Source: CAD feature listing. Evaluate the final solid. Frame: model axes, mm. A direction names the side the tool comes from. Round coordinates to 2 decimals unless told otherwise and drop trailing zeros. Write each loop counter-clockwise with the first axis right and the second up, starting at its lowest first coordinate (ties: lowest second). Pieces come first, ordered by that corner, then holes. Notation, with made-up numbers: M 5,68 L 47,68 A25 ccw 47,81 Z; hole C 32.25,8.5 d5. An arc over 180 degrees is marked long. Put each result on its own line as item: value. Start each with the question number.
```python
from build123d import *
from OCP.BRepFilletAPI import BRepFilletAPI_MakeChamfer

# Parameters (mm, degrees)
ESQUISSE1_W             = 62
ESQUISSE1_H             = 42
BOSS_EXTRU_1_DEPTH      = 15
ESQUISSE2_R             = 2.1
ESQUISSE2_R_2           = 12.5
ESQUISSE2_R_3           = 1.7
ENL_V_MAT_EXTRU_1_DEPTH = 41.33608806
ESQUISSE4_R             = 4.5
ENL_V_MAT_EXTRU_2_DEPTH = 10
SKETCH1_W               = 20
SKETCH1_H               = 42
CUT_EXTRUDE1_DEPTH      = 41.33608806
SKETCH2_W               = 15
SKETCH2_H               = 42
BOSS_EXTRUDE1_DEPTH     = 40
CUT_EXTRUDE2_DEPTH      = 68.749538744
SKETCH7_W               = 38
SKETCH7_H               = 20
CUT_EXTRUDE3_DEPTH      = 7
SKETCH9_R               = 2.1
CUT_EXTRUDE4_DEPTH      = 56.731499172
CHAMFER1_SIZE           = 38
CHAMFER1_SIZE2          = 11
SKETCH10_W              = 8
SKETCH10_H              = 24.631578948
CUT_EXTRUDE5_DEPTH      = 58.15767665
FILLET2_START           = -1
FILLET2_DEPTH           = 17
FILLET2_START_2         = -22
FILLET2_2_DEPTH         = 44
FILLET4_R               = 2
FILLET5_R               = 1


with BuildPart() as part:
    # Esquisse1 → Boss.-Extru.1 (new body)
    with BuildSketch(Plane.XY):
        Rectangle(ESQUISSE1_W, ESQUISSE1_H)
    extrude(amount=BOSS_EXTRU_1_DEPTH)

    # Esquisse2 → Enlèv. mat.-Extru.1 (cut, through all)
    with BuildSketch(Plane.XY.offset(15)):
        with Locations((21, 11)):
            Circle(ESQUISSE2_R)
        with Locations((21, -11)):
            Circle(ESQUISSE2_R)
        with Locations((-10, 0)):
            Circle(ESQUISSE2_R_2)
        with Locations((-25.5, 15.5)):
            Circle(ESQUISSE2_R_3)
        with Locations((5.5, 15.5)):
            Circle(ESQUISSE2_R_3)
        with Locations((5.5, -15.5)):
            Circle(ESQUISSE2_R_3)
        with Locations((-25.5, -15.5)):
            Circle(ESQUISSE2_R_3)
    extrude(amount=-ENL_V_MAT_EXTRU_1_DEPTH, mode=Mode.SUBTRACT)

    # Esquisse4 → Enlèv. mat.-Extru.2 (cut)
    with BuildSketch(Plane.XY.offset(15)):
        with Locations((-25.5, 15.5)):
            Circle(ESQUISSE4_R)
        with Locations((-25.5, -15.5)):
            Circle(ESQUISSE4_R)
        with Locations((5.5, -15.5)):
            Circle(ESQUISSE4_R)
        with Locations((5.5, 15.5)):
            Circle(ESQUISSE4_R)
    extrude(amount=-ENL_V_MAT_EXTRU_2_DEPTH, mode=Mode.SUBTRACT)

    # Sketch1 → Cut-Extrude1 (cut, through all)
    with BuildSketch(Plane.XY.offset(15)):
        with Locations((21, 0)):
            Rectangle(SKETCH1_W, SKETCH1_H)
    extrude(amount=-CUT_EXTRUDE1_DEPTH, mode=Mode.SUBTRACT)

    # Sketch2 → Boss-Extrude1 (add)
    with BuildSketch(Plane(origin=(11, 0, 0), x_dir=(0, 0, -1), z_dir=(1, 0, 0))):
        with Locations((-7.5, 0)):
            Rectangle(SKETCH2_W, SKETCH2_H)
    extrude(amount=BOSS_EXTRUDE1_DEPTH)

    # Sketch6 → Cut-Extrude2 (cut, through all)
    with BuildSketch(Plane.XZ.offset(21)):
        Polygon((-31, 8), (-31, 15), (13, 15), align=None)
    extrude(amount=-CUT_EXTRUDE2_DEPTH, mode=Mode.SUBTRACT)

    # Sketch7 → Cut-Extrude3 (cut)
    with BuildSketch(Plane.XY.offset(15)):
        with Locations((32, 0)):
            Rectangle(SKETCH7_W, SKETCH7_H)
    extrude(amount=-CUT_EXTRUDE3_DEPTH, mode=Mode.SUBTRACT)

    # Sketch9 → Cut-Extrude4 (cut, through all)
    with BuildSketch(Plane.XY.offset(8)):
        with Locations((21, 0)):
            Circle(SKETCH9_R)
        with Locations((35, 0)):
            Circle(SKETCH9_R)
    extrude(amount=-CUT_EXTRUDE4_DEPTH, mode=Mode.SUBTRACT)

    # Chamfer1: one chamfer whose edges measure the first distance from different faces: ONE call of the kernel's chamfer builder (chamfer() names one face for all edges)
    chamfer1_edges_1 = [part.edges().sort_by_distance(p)[0] for p in [
        (51, 21, 7.5),
    ]]
    chamfer1_side_1 = [part.faces().sort_by_distance(p)[0] for p in [
        (13.76889715, 21, 6.760532838),
    ]]
    chamfer1_edges_2 = [part.edges().sort_by_distance(p)[0] for p in [
        (51, -21, 7.5),
    ]]
    chamfer1_side_2 = [part.faces().sort_by_distance(p)[0] for p in [
        (13.76889715, -21, 6.760532838),
    ]]
    chamfer1 = BRepFilletAPI_MakeChamfer(part.part.solid().wrapped)
    for e in chamfer1_edges_1:
        chamfer1.Add(CHAMFER1_SIZE, CHAMFER1_SIZE2, e.wrapped, chamfer1_side_1[0].wrapped)  # the first distance lies on this face
    for e in chamfer1_edges_2:
        chamfer1.Add(CHAMFER1_SIZE, CHAMFER1_SIZE2, e.wrapped, chamfer1_side_2[0].wrapped)  # the first distance lies on this face
    add(Compound.cast(chamfer1.Shape()), mode=Mode.REPLACE)

    # Sketch10 → Cut-Extrude5 (cut, through all)
    with BuildSketch(Plane(origin=(0, 0, 0), x_dir=(-1, 0, 0), z_dir=(0, 0, -1))):
        with Locations((-47, 0)):
            Rectangle(SKETCH10_W, SKETCH10_H)
    extrude(amount=-CUT_EXTRUDE5_DEPTH, mode=Mode.SUBTRACT)

    # Fillet2: read off the stored shape, not the designer's step
    # Fillet2 outline → Fillet2 (cut)
    with BuildSketch(Plane.XY.offset(FILLET2_START)):
        with BuildLine():
            Line((13, 21), (10.163489291, 21))
            ThreePointArc((10.163489291, 21), (12.9718958, 20.801839634), (15.724650822, 20.211285288))
            Line((15.724650822, 20.211285288), (13, 21))
        make_face()
        with BuildLine():
            ThreePointArc((15.724650822, -20.211285288), (12.9718958, -20.801839634), (10.163489291, -21))
            Line((10.163489291, -21), (13, -21))
            Line((13, -21), (15.724650822, -20.211285288))
        make_face()
    extrude(amount=FILLET2_DEPTH, mode=Mode.SUBTRACT)

    # Fillet2 2 outline → Fillet2 2 (cut)
    with BuildSketch(Plane(origin=(0, 0, 0), x_dir=(1, 0, 0), z_dir=(0, 1, 0)).offset(FILLET2_START_2)):
        with BuildLine():
            Line((11.438667082, -14.751606127), (13, -15))
            Line((13, -15), (14.580968057, -15))
            ThreePointArc((14.580968057, -15), (13.004916429, -14.937804826), (11.438667082, -14.751606127))
        make_face()
    extrude(amount=FILLET2_2_DEPTH, mode=Mode.SUBTRACT)

    # Fillet4
    fillet4_edges = [part.edges().sort_by_distance(p)[0] for p in [
        (-31, 21, 4),
        (-31, -21, 4),
    ]]
    fillet(fillet4_edges, radius=FILLET4_R)

    # Fillet5
    fillet5_edges = [part.edges().sort_by_distance(p)[0] for p in [
        (43, -10, 11.5),
        (43, 10, 11.5),
        (43, 12.315789474, 7.5),
        (43, -12.315789474, 7.5),
    ]]
    fillet(fillet5_edges, radius=FILLET5_R)


solid = part.part
```
(1) Section query D-D (y = -15.5). Return loops of the section in (x, z), and give its area (3 significant figures).
(2) Section query A-A (y = 4). Return loops of the section in (x, z).
(3) Ray query, line 1 along Y through (x, z) = (-25.5, 1.9); line 2 along Y through (x, z) = (16.5, 14.5); line 3 along X through (y, z) = (7, 4.25). Return the intervals inside material, ascending.
(4) Section query C-C (z = 3.25). Return loops of the section in (x, y), and give its area (3 significant figures).
(5) Pull-direction query (Y, two-part tool) for faces 4 (the flat face through (25, 14, 15)), 5 (the flat face through (29.187, 16.314, 7.605)), 6 (the flat face through (29.187, -16.314, 7.605)), 7 (the flat face through (13, 0, 12)); classes: +Y half, -Y half, draft (parallel to the pull), parting line (faces both ways), or undercut.
(6) Access query for faces 1 (the flat face through (-31, 0, 4)), 2 (the flat face through (5.4, 13.6, 5)), 3 (the flat face through (27, 10, 12)). Directions: +Z, -Z, +X, -X, +Y, -Y. A direction counts if a zero-diameter tool reaches every point of the face in a straight line with its end or side. Return the directions, or none.
(7) Contact query for flat-ended pins moving along their axis: P1, Ø5.5, axis at x = -25.5, y = -15.5, coming from the +Z side; P2, Ø8, axis at y = 1, z = 11, coming from the -X side; P3, Ø10, axis at x = 7, y = -14, coming from the +Z side; P4, Ø2, axis at x = 25.5, z = 6.5, coming from the -Y side. Output: stop coordinate, or through.
(8) Section query B-B (x = 35). Return loops of the section in (y, z), and give its area (3 significant figures).
Entries:
1. outline: M -31,0 L -27.2,0 L -27.2,5 L -30,5 L -30,8.16 L -31,8 Z; M -23.8,0 L 3.8,0 L 3.8,5 L 1,5 L 1,13.09 L -21,9.59 L -21,5 L -23.8,5 Z; M 7.2,0 L 32,0 L 32,15 L 14.58,15 A20 ccw 11.44,14.75 L 10,14.52 L 10,5 L 7.2,5 Z
1. area: 643 mm2
2. outline: M -31,0 L -21.84,0 L -21.84,9.46 L -31,8 Z; M 1.84,0 L 43,0 L 43,8 L 13,8 L 13,14.94 A20 ccw 11.44,14.75 L 1.84,13.22 Z
3. line 1: -21 to -17.2, -13.8 to 13.8, 17.2 to 21
3. line 2: -19.99 to -10, 10 to 19.99
3. line 3: -31 to -20.36, 0.36 to 43
4. outline: M -31,-19 A2 ccw -29,-21 L 10.16,-21 A20 ccw 15.72,-20.21 L 42.28,-12.52 A1 ccw 43,-11.56 L 43,11.56 A1 ccw 42.28,12.52 L 15.72,20.21 A20 ccw 10.16,21 L -29,21 A2 ccw -31,19 Z; hole C -25.5,-15.5 d3.4; hole C -25.5,15.5 d3.4; hole C -10,0 d25; hole C 5.5,-15.5 d3.4; hole C 5.5,15.5 d3.4; hole C 21,0 d4.2; hole C 35,0 d4.2
4. area: 2,290 mm2
5. face 4: draft
5. face 5: +Y half
5. face 6: -Y half
5. face 7: undercut
6. face 1: +Z, -Z, -X, +Y, -Y
6. face 2: +Z
6. face 3: +Z, +X
7. P1: z = 5
7. P2: x = -31
7. P3: z = 14.83
7. P4: y = -17.67
8. outline: M -14.63,0 L -2.1,0 L -2.1,8 L -10,8 L -10,15 L -14.63,15 Z; M 2.1,0 L 14.63,0 L 14.63,15 L 10,15 L 10,8 L 2.1,8 Z
8. area: 265 mm2
